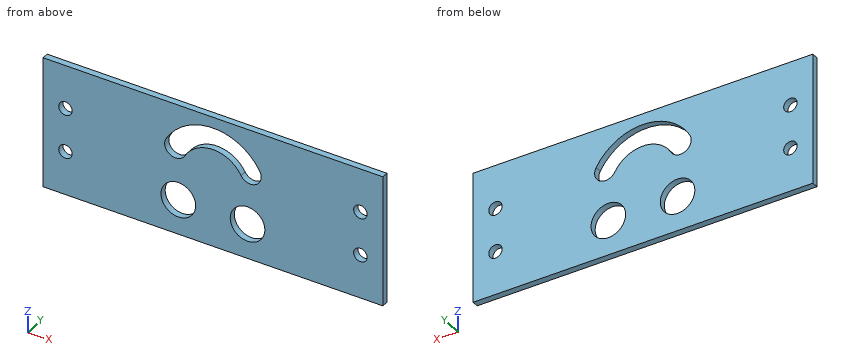
Autodesk Inventor part; units mm, degrees
ref_plane "YZ Plane" through (0, 0, 0) normal (1, 0, 0) x (0, 1, 0)
ref_plane "XZ Plane" through (0, 0, 0) normal (0, 1, 0) x (-1, 0, 0)
ref_plane "XY Plane" through (0, 0, 0) normal (0, 0, 1) x (1, 0, 0)
sketch "Sketch1" plane through (0, 0, 0) normal (0, 1, 0) x (-1, 0, 0)
  line L0 (20.6396, 0) -> (20.6396, -30)
  line L1 (57.9189, -30) -> (57.9189, 0)
  arc A0 (50.1046, -8.75) -> (28.454, -8.75) centre (39.2793, -15) ccw
  arc A1 (28.454, -8.75) -> (32.7841, -11.25) centre (30.619, -10) ccw
  arc A2 (45.7745, -11.25) -> (32.7841, -11.25) centre (39.2793, -15) ccw
  arc A3 (45.7745, -11.25) -> (50.1046, -8.75) centre (47.9395, -10) ccw
  circle A4 centre (47.2793, -22) radius 4
  circle A5 centre (31.2793, -22) radius 4
  circle A6 centre (73.3686, -10) radius 1.55
  circle A7 centre (5.19, -10) radius 1.55
  circle A8 centre (73.3686, -20) radius 1.55
  circle A9 centre (5.19, -20) radius 1.55
  line L2 (0, -30) -> (0, 0)
  line L3 (78.5586, -30) -> (0, -30)
  line L4 (0, 0) -> (78.5586, 0)
  line L5 (78.5586, 0) -> (78.5586, -30)
  line L6 (58.3686, 0) -> (58.3686, -30)
  line L7 (57.4693, -30) -> (57.4693, 0)
  line L8 (21.0893, 0) -> (21.0893, -30)
  line L9 (20.19, -30) -> (20.19, 0)
extrude "Extrusion1" add sketch "Sketch1" against normal blind 1.5
properties part number "Head2"
Part model, mm, in its own coordinate system. Give positions to 0.01 mm unless a question says otherwise; leave off trailing zeros. Write each loop counter-clockwise with the first axis right and the second up, starting at its lowest first coordinate (ties: lowest second). Pieces come first, ordered by that corner, then holes. Notation, with made-up numbers: (79, 71.5) -> (127, 71.5) arc R31 ccw to (127, 98.5) -> close; hole circle Ø1 at (-13, -24). An arc over 180 degrees is marked (long way). Put each result on its own line as item: value. Start each with the question number.
Item 1: Cut at C-C (z = -25.25). List the corners of the cut face in (x, y).
Item 2: Cut at B-B (y = -0.4). List the corners of the cut face in (x, z), then the cut area to 3 significant figures.
Item 3: Cut at A-A (x = -5.19). List the corners of the cut face in (y, z).
Item 4: Cut at D-D (z = -10). List the corners of the cut face in (x, y), then the cut area to 3 significant figures.
Item 5: Wall check: L1, parallel to Z at x = -5.19, y = -1.2; L2, parallel to Z at x = -34, y = -1.15; L3, parallel to X at y = -0.8, z = -24.5. Give the ranges that are in metal, low to high. Write a range as [from, to].
Answer list:
1. outline: (-78.56, -1.5) -> (-49.61, -1.5) -> (-49.61, 0) -> (-78.56, 0) -> close; (-44.95, -1.5) -> (-33.61, -1.5) -> (-33.61, 0) -> (-44.95, 0) -> close; (-28.95, -1.5) -> (0, -1.5) -> (0, 0) -> (-28.95, 0) -> close
2. outline: (-78.56, -30) -> (0, -30) -> (0, 0) -> (-78.56, 0) -> close; hole circle Ø3.1 at (-73.37, -20); hole circle Ø3.1 at (-73.37, -10); hole circle Ø8 at (-47.28, -22); hole (-50.1, -8.75) arc R2.5 ccw to (-45.77, -11.25) arc R7.5 cw to (-32.78, -11.25) arc R2.5 ccw to (-28.45, -8.75) arc R12.5 ccw to start; hole circle Ø8 at (-31.28, -22); hole circle Ø3.1 at (-5.19, -20); hole circle Ø3.1 at (-5.19, -10)
2. area: 2,100 mm2
3. outline: (-1.5, -30) -> (0, -30) -> (0, -21.55) -> (-1.5, -21.55) -> close; (-1.5, -18.45) -> (0, -18.45) -> (0, -11.55) -> (-1.5, -11.55) -> close; (-1.5, -8.45) -> (0, -8.45) -> (0, 0) -> (-1.5, 0) -> close
4. outline: (-78.56, -1.5) -> (-74.92, -1.5) -> (-74.92, 0) -> (-78.56, 0) -> close; (-71.82, -1.5) -> (-50.44, -1.5) -> (-50.44, 0) -> (-71.82, 0) -> close; (-44.87, -1.5) -> (-33.69, -1.5) -> (-33.69, 0) -> (-44.87, 0) -> close; (-28.12, -1.5) -> (-6.74, -1.5) -> (-6.74, 0) -> (-28.12, 0) -> close; (-3.64, -1.5) -> (0, -1.5) -> (0, 0) -> (-3.64, 0) -> close
4. area: 91.8 mm2
5. L1: z = [-30, -21.55], [-18.45, -11.55], [-8.45, 0]
5. L2: z = [-30, -24.93], [-19.07, -9.67], [-3.67, 0]
5. L3: x = [-78.56, -50.4], [-44.16, -34.4], [-28.16, 0]
